Can you work these out from the model? Positions are in its coordinate system, mm. Give positions to 0.01 mm unless a question says otherwise; leave off trailing zeros. Order: outer loops, then holes, each group sorted by start corner. A loop starts at its lowest first (then second) coordinate and runs counter-clockwise, first axis right, second up. Notation, with made-up numbers: (-31, 53) - (-11, 53) arc R18 cw to (-11, 67) - close; hole circle Ø2 at (-36, 70). An arc over 180 degrees is marked (long way). Write each question's results on one line, items separated by ' | '. Start each with the question number.
Autodesk Inventor part; units mm, degrees
ref_plane "YZ Plane" through (0, 0, 0) normal (1, 0, 0) x (0, 1, 0)
ref_plane "XZ Plane" through (0, 0, 0) normal (0, 1, 0) x (-1, 0, 0)
ref_plane "XY Plane" through (0, 0, 0) normal (0, 0, 1) x (1, 0, 0)
sketch "Sketch1" plane through (0, 0, 0) normal (0, 1, 0) x (-1, 0, 0)
  circle A0 centre (0, 0) radius 267
  circle A1 centre (0, 0) radius 335
  line L0 (335, 0) -> (267, 0)
  line L1 (-267, 0) -> (-335, 0)
  line L2 (0, 267) -> (0, 335)
  point P0 (301, 0)
  point P1 (-301, 0)
  point P2 (0, 301)
  dimension "d1" = 670
  dimension "d4" = 534
extrude "Extrusion1" add sketch "Sketch1" along normal blind 8 contours L0 A1 L1 A0 | A0 L2 A1 L0 | A0 L1 A1 L2
sketch "Sketch2" plane through (0, 0, 0) normal (0, -1, 0) x (1, 0, 0)
  line L0 (0, 0) -> (0, 310) construction
  line L1 (0, 0) -> (48.4947, 306.1834) construction
  circle A0 centre (0, 0) radius 310 construction
  dimension "d14" = 620
  dimension "d15" = 9
hole "Hole1" at (48.4947, 0, 306.1834) direction (0, 1, 0) diameter 26 end through all
pattern_circular "Circular Pattern2" count 20 over 360 about axis through (0, -10, 0) along (0, 1, 0) of "Hole1"
equation "\"d2\" = Thickness"
equation "\"d21\" = Thickness"
equation "\"BendRadius\" = Thickness"
equation "\"BendReliefWidth\" = Thickness"
equation "\"BendReliefDepth\" = 0.5 * Thickness"
equation "\"CornerReliefSize\" = 4 * Thickness"
equation "\"MinimumRemnant\" = 2 * Thickness"
equation "\"TransitionRadius\" = BendRadius"
equation "\"JacobiRadiusSize\" = BendRadius"
equation "\"GapSize\" = Thickness"
equation "\"d8\" = Thickness"
properties part number "!!PRS 9512 accses hatch flangeipt_D1200"
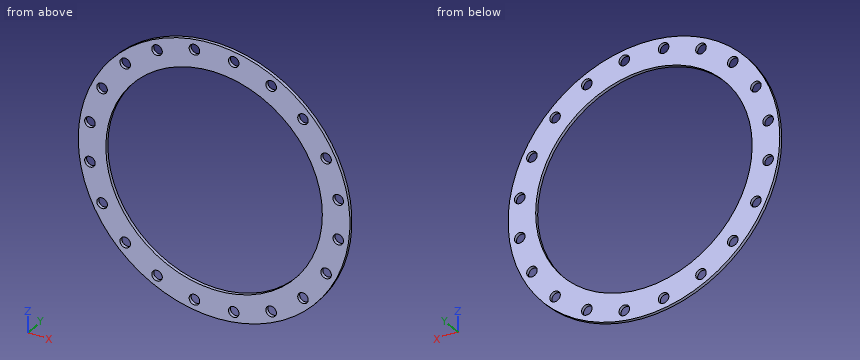
Q1. If we section it at A-A (x = 0): Please give me the cut outline in (y, z), plus the area to 3 significant figures.
Q2. If I drill on probe 1 along Z at (x, y) = (307, 5); probe 2 along Z at (x, y) = (-53, 1.5); probe 3 along X at (y, z) = (0.5, -222), over which ranges is the centre line in solid material (lowest first)? Write a range as from..to.
Q3. If we section it at B-B (z = 0): Please give me the cut outline in (x, y).
Q4. Will these pins go through, and if not, where does the flat tip stop? P1, Ø1, axis at y = 6, z = 27.5, coming from the +X side; P2, Ø2, axis at y = 7, z = 158.5, coming from the +X side; P3, Ø1, axis at x = 188.5, y = 4.5, coming from the +Z side.
Findings below:
1) outline: (0, -335) - (8, -335) - (8, -267) - (0, -267) - close; (0, 267) - (8, 267) - (8, 335) - (0, 335) - close | area: 1,090 mm2
2) probe 1: z = -134.07..-61.47, -35.52..35.52, 61.47..134.07 | probe 2: z = -330.78..-318.38, -293.99..-261.69, 261.69..293.99, 318.38..330.78 | probe 3: x = -250.88..-231.9, -206.51..-148.34, 148.34..206.51, 231.9..250.88
3) outline: (-335, 0) - (-267, 0) - (-267, 8) - (-335, 8) - close; (267, 0) - (335, 0) - (335, 8) - (267, 8) - close
4) P1: stops at x = 333.91 | P2: stops at x = 295.67 | P3: stops at z = 277.27
